Geometry: final body of the model. Coordinates: model frame, mm. Face numbers are marked on the shaded views. A direction names the side the tool comes from. Give positions to 0.01 mm unless a question says otherwise; leave off trailing zeros. Write each loop counter-clockwise with the first axis right and the second up, starting at its lowest first coordinate (ties: lowest second). Pieces come first, ordered by that corner, then holes. Notation, with made-up numbers: (2, -10) -> (25, -10) arc R29 cw to (25, 12) -> close; hole circle Ø3 at (74.25, 73). An arc over 180 degrees is marked (long way). Answer as a JSON object with one key per item and string values.
Autodesk Inventor part; units mm, degrees
ref_plane "YZ Plane" through (0, 0, 0) normal (1, 0, 0) x (0, 1, 0)
ref_plane "XZ Plane" through (0, 0, 0) normal (0, 1, 0) x (-1, 0, 0)
ref_plane "XY Plane" through (0, 0, 0) normal (0, 0, 1) x (1, 0, 0)
sketch "Sketch1" plane through (0, 0, 0) normal (0, 0, 1) x (1, 0, 0)
  line L0 (92.558, -5.5266) -> (88.4016, -5.5266)
  line L1 (88.4016, -5.5266) -> (88.4016, -2.3241)
  line L2 (88.4016, -2.3241) -> (92.558, -2.3241)
  line L3 (92.558, -2.3241) -> (92.558, -5.5266)
  line L4 (91.8766, -5.0496) -> (88.9467, -5.0496)
  line L5 (88.9467, -5.0496) -> (88.9467, -2.8011)
  line L6 (88.9467, -2.8011) -> (91.8766, -2.8011)
  line L7 (91.8766, -2.8011) -> (91.8766, -5.0496)
  point P0 (0, 0)
extrude "Extrusion1" add sketch "Sketch1" along normal blind 4
sketch "Sketch3" plane through (92.558, -5.5266, 0) normal (1, 0, 0) x (0, 0, -1)
  line L0 (-4, 0) -> (-4, 3.2025)
  line L1 (0, 3.2025) -> (0, 0)
  point P0 (0, 5.5266)
sketch "Sketch4" plane through (88.9467, -5.0496, 0) normal (1, 0, 0) x (0, 0, -1)
  line L0 (0, 2.7255) -> (0, -0.477)
  line L1 (0, -0.477) -> (4.8951, -0.7122)
  line L2 (4.8951, -0.7122) -> (7.0077, -0.8137)
  line L3 (7.0077, -0.8137) -> (7.9085, -0.5009)
  line L4 (7.9085, -0.5009) -> (8.2533, 0.0718)
  line L5 (8.2533, 0.0718) -> (8.3068, 1.1847)
  line L6 (8.3068, 1.1847) -> (8.0262, 1.993)
  line L7 (8.0262, 1.993) -> (7.0621, 2.6005)
  line L8 (7.0621, 2.6005) -> (3.5876, 2.6005)
  line L9 (3.5876, 2.6005) -> (-0.3844, 2.3008)
  line L10 (-0.3844, 2.3008) -> (-5.3135, 2.6005)
  line L11 (-5.3135, 2.6005) -> (-8.9119, 3.2451)
  line L12 (-8.9119, 3.2451) -> (-12.4072, 3.8713)
  line L13 (-12.4072, 3.8713) -> (-12.517, 3.2581)
  line L14 (-12.517, 3.2581) -> (-7.6517, 2.3865)
  line L15 (-7.6517, 2.3865) -> (-4.6985, 1.9752)
  line L16 (-4.6985, 1.9752) -> (-0.7689, 1.7864)
  line L17 (-0.7689, 1.7864) -> (2.2504, 2.0142)
  line L18 (2.2504, 2.0142) -> (6.5148, 1.7549)
  line L19 (6.5148, 1.7549) -> (7.1634, 1.7155)
  line L20 (7.1634, 1.7155) -> (7.6433, 1.4131)
  line L21 (7.6433, 1.4131) -> (7.6418, 1.3822)
  line L22 (7.6418, 1.3822) -> (7.5978, 0.465)
  line L23 (7.5978, 0.465) -> (7.5874, 0.25)
  line L24 (7.5874, 0.25) -> (6.9873, 0.0994)
  line L25 (6.9873, 0.0994) -> (5.6698, 0)
  line L26 (0, 0) -> (-4, 0)
  line L27 (5.6698, 0) -> (0, 0)
  line L28 (0, 0) -> (0, -0.477)
  point P0 (0, 5.0496)
extrude "Extrusion2" add sketch "Sketch4" along normal blind 2.5 contours L27 L25 L24 L23 L22 L21 L20 L19 L18 L17 L0 L9 L8 L7 L6 L5 L4 L3 L2 L1 | L17 L16 L15 L14 L13 L12 L11 L10 L9 L0
sketch "Sketch5" plane through (88.9467, -5.0496, 4) normal (1, 0, 0) x (0, 0, -1)
  line L0 (4, 0) -> (0, 0)
  line L1 (0, 0) -> (0.9929, 0)
  line L2 (0.9929, 0) -> (1.9546, 1.1114)
  line L3 (1.9546, 1.1114) -> (1.4737, 1.2793)
  line L4 (0, 0) -> (0, 1.9416)
  line L5 (1.4737, 1.2793) -> (0, 0)
  point P0 (4, 5.0496)
extrude "Extrusion3" add sketch "Sketch5" along normal blind 2
properties part number "Ziptie"
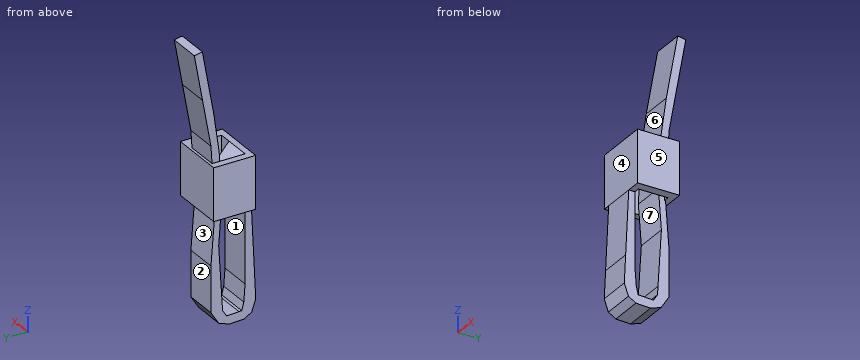
Q1. Cut plane B-B (z = 1). Return the cut outline in (x, y), and give its area (3 significant figures).
Values:
{"outline": "(88.4, -5.53) -> (92.56, -5.53) -> (92.56, -2.32) -> (88.4, -2.32) -> close; hole (88.95, -5.05) -> (91.88, -5.05) -> (91.88, -2.8) -> (91.45, -2.8) -> (91.45, -3.25) -> (88.95, -3.25) -> close", "area": "7.85 mm²"}
Q2. First-contact query: P1, Ø0.9, axis at x = 91, z = -1.5, coming from the +Y side; P2, Ø1.5, axis at x = 92, y = -5, coming from the +Z side; P3, Ø0.6, axis at y = -2, z = 10, coming from the -X side. Flat tips, straight axial feed; report the tip coordinate or a pass-through.
Values:
{"P1": "y = -2.57", "P2": "z = 4", "P3": "x = 88.95"}
Q3. Set-up query: the marked faces 1, 2, 3 and 4. Return all of +Z, -Z, +X, -X, +Y, -Y with unobstructed straight access to the full face (end or side cutting, diameter ignored); none if empty.
Values:
{"face 1": "none", "face 2": "-Z, +X, -X, +Y", "face 3": "+X, -X, +Y", "face 4": "+Z, +X, -X, -Y"}
Q4. Cut plane C-C (z = -3.25). Return the cut outline in (x, y).
Values:
{"outline": "(88.95, -5.68) -> (91.45, -5.68) -> (91.45, -5.05) -> (88.95, -5.05) -> close; (88.95, -3.1) -> (91.45, -3.1) -> (91.45, -2.47) -> (88.95, -2.47) -> close"}
Q5. Material intervals for L1, parallel to X at y = -3.2, z = 0.75; L2, parallel to Y at x = 90.65, z = -7; L3, parallel to Y at x = 89.8, z = -0.75, sorted ascending. Write a range as from..to.
Values:
{"L1": "88.4..91.45, 91.88..92.56", "L2": "-5.86..-4.95, -3.32..-2.45", "L3": "-5.56..-5.05, -3.15..-2.66"}
Q6. Mould query, pull axis Z, two halves, no side actions, for the marked faces 5, 6 and 7. Classes: pulls with the +Z half, pulls with the -Z half, needs draft (parallel to the pull), parting line crosses it, or undercut.
Values:
{"face 5": "needs draft", "face 6": "pulls with the +Z half", "face 7": "undercut"}
